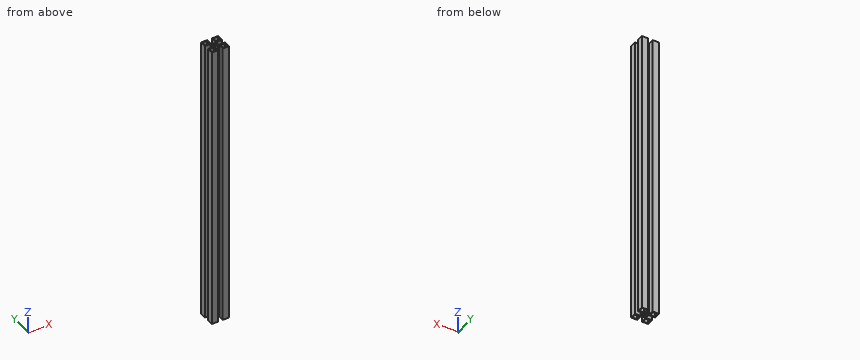
```python
from build123d import *

# Parameters (mm, degrees)
SKETCH_W      = 30.196043
SKETCH_H      = 30.018427
PAD_DEPTH     = 500
SKETCH001_R   = 2.124228
SKETCH001_W   = 8.189246
SKETCH001_H   = 8.189245
SKETCH001_W_2 = 8.203447
SKETCH001_H_2 = 7.852266
SKETCH001_W_3 = 8.321901
SKETCH001_H_3 = 8.144941
SKETCH001_W_4 = 8.345211
SKETCH001_H_4 = 8.02151
POCKET_DEPTH  = 500


with BuildPart() as part:
    # Sketch → Pad (new body)
    with BuildSketch(Plane.XY):
        with Locations((15.098021, 15.009213)):
            Rectangle(SKETCH_W, SKETCH_H)
    extrude(amount=PAD_DEPTH)

    # Sketch001 → Pocket (cut)
    with BuildSketch(Plane.XY.offset(500)):
        with Locations((14.887853, 15.18749)):
            Circle(SKETCH001_R)
        with Locations((5.35938, 5.342074)):
            Rectangle(SKETCH001_W, SKETCH001_H)
        with Locations((24.923182, 5.242986)):
            Rectangle(SKETCH001_W_2, SKETCH001_H_2)
        with Locations((24.643347, 24.908541)):
            Rectangle(SKETCH001_W_3, SKETCH001_H_3)
        with Locations((5.274876, 24.623256)):
            Rectangle(SKETCH001_W_4, SKETCH001_H_4)
        Polygon((19.170053, 9.228496), (19.170053, -1.667364), (10.77261, -1.667364), (10.77261, 9.228496), (12.854619, 11.102304), (17.088041, 11.102304), align=None)
        Polygon((32.078522, 11.310507), (20.835663, 11.310507), (17.990246, 13.253717), (17.990246, 16.584934), (20.835663, 18.875151), (32.078522, 18.875151), align=None)
        Polygon((11.189011, 31.922419), (19.239456, 31.922419), (19.239456, 20.401957), (16.46344, 18.042343), (13.20162, 18.042343), (11.189011, 20.401957), align=None)
        Polygon((-4.773074, 19.15275), (9.6622, 19.15275), (11.813614, 16.654335), (11.813614, 13.045515), (9.6622, 10.963505), (-4.773074, 10.963505), align=None)
    extrude(amount=-POCKET_DEPTH, mode=Mode.SUBTRACT)


solid = part.part
```
Geometry: final body of the model. Coordinates: model frame, mm. Coordinates: 2 decimals unless noted, no trailing zeros. Use a Markdown table: item, result. Add a question column.
(1) Line query: line 1 along X through (y, z) = (6.5, 95.5); line 2 along Y through (x, z) = (2.5, 303); line 3 along Y through (x, z) = (24, 289). Output: solid intervals per line, ascending.
(2) Pin query (flat end, axial travel): pin 1 Ø4 at (x, y) = (14.89, 15.19) entering from -Z (3 decimals); pin 2 Ø3 at (y, z) = (14, 231) entering from -X. Return the tip coordinate at first contact, or that it passes through.
(3) Section query A-A, the plane z = 432. State how many separate pieces and enclosed holes the cut face has, plus the area to 3 significant figures.
Answer:
| question | item | result |
|---|---|---|
| 1 | line 1 | x = 0 to 1.26, 9.45 to 10.77, 19.17 to 20.82, 29.02 to 30.2 |
| 1 | line 2 | y = 0 to 1.25, 9.44 to 10.96, 19.15 to 20.61, 28.63 to 30.02 |
| 1 | line 3 | y = 0 to 1.32, 9.17 to 11.31, 18.88 to 20.84, 28.98 to 30.02 |
| 2 | pin 1 | passes through |
| 2 | pin 2 | stops at x = 11.25 |
| 3 | separate pieces | 1 |
| 3 | enclosed holes | 5 |
| 3 | area | 268 mm^2 |
